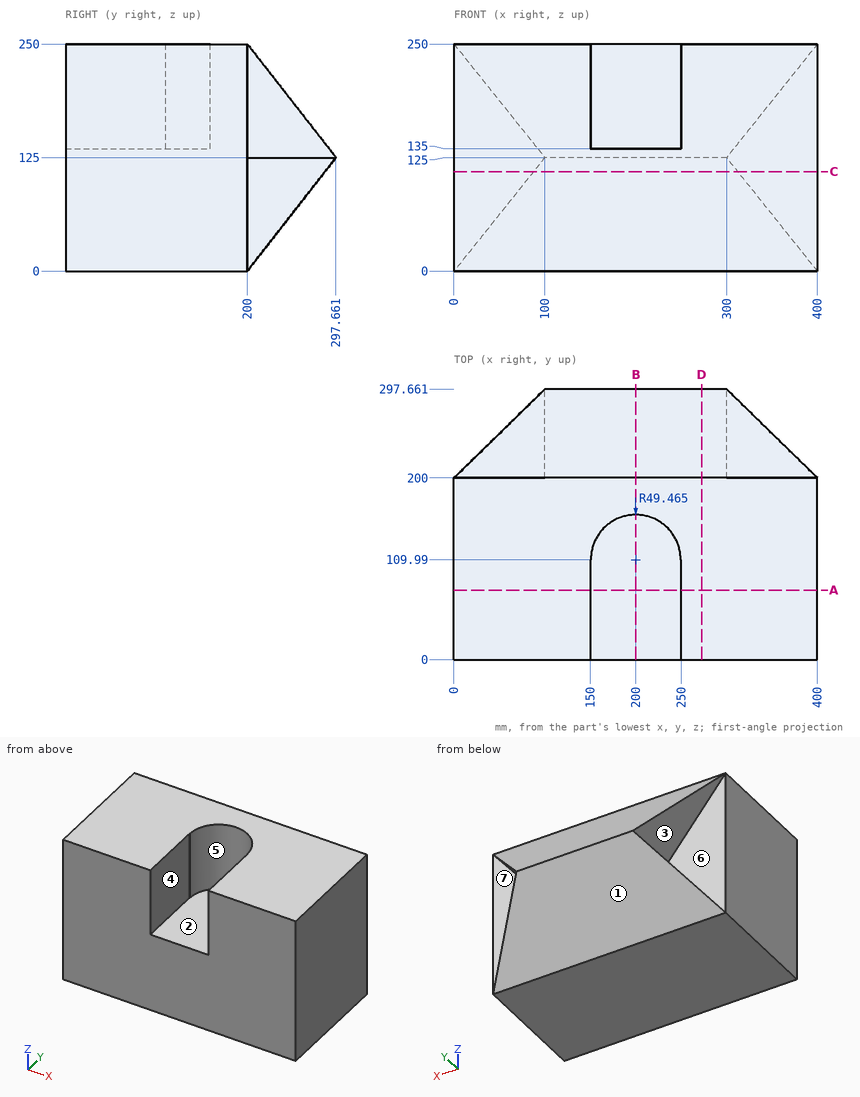
Part print with two shaded views. Sizes in mm from the minimum x, y, z corner. A direction names the side the tool comes from. Round coordinates to 2 decimals unless told otherwise and drop trailing zeros. Order: outer loops, then holes, each group sorted by start corner. A loop starts at its lowest first (then second) coordinate and runs counter-clockwise, first axis right, second up. Notation, with made-up numbers: (24.5, 48.5) - (83.5, 48.5) arc R19 cw to (83.5, 63.5) - close; hole circle Ø3 at (76, -11). An arc over 180 degrees is marked (long way). Answer as CSV lines item,"result". Start each with the question number.
1. Saw through at D-D, the plane x = 272.5. Write the cut outline in (y, z), and give its area (3 significant figures).
2. Saw through at B-B, the plane x = 200. Write the cut outline in (y, z) (1 decimal).
3. Tool access for the marked faces 5, 6 and 7: list every direction of +Z, -Z, +X, -X, +Y, -Y with a clear straight run to the whole face (end or side of a thin tool).
4. Pin check, flat tips, straight feed: pin 1 (5 mm diameter, centred on y = 230, z = 149, fed in from -X); pin 2 (3 mm diameter, centred on x = 161, y = 259, fed in from -Z); pin 3 (3 mm diameter, centred on x = 238.5, z = 121.5, fed in from +Y). Stop position of each tip, or through.
5. Drill centre lines: L1, parallel to X at y = 65.5, z = 187; L2, parallel to Z at x = 84, y = 220; L3, parallel to Y at x = 20.5, z = 221. Where is each one in solid material? Low to high. Write a range as [from, to].
6. Saw through at A-A, the plane y = 76.5. Write the cut outline in (x, z), and give its area (3 significant figures).
7. Saw through at C-C, the plane z = 109.5. Write the cut outline in (x, y).
8. Pull direction X, two halves, no side cores. Call the marked faces 1, 2, 3 and 4: +X half, -X half, draft (parallel to the pull), parting line (faces both ways), or undercut.
Model answer:
1,outline,"(0, 0) - (200, 0) - (297.66, 125) - (200, 250) - (0, 250) - close"
1,area,"62,200 mm²"
2,outline,"(0, 0) - (200, 0) - (297.7, 125) - (200, 250) - (159.5, 250) - (159.5, 135) - (0, 135) - close"
3,face 5,"+Z, -Y"
3,face 6,"-X, +Y"
3,face 7,"+X, +Y"
4,pin 1,"stops at x = 78.8"
4,pin 2,"stops at z = 73.6"
4,pin 3,"stops at y = 296.1"
5,L1,"x = [0, 150], [250, 400]"
5,L2,"z = [25.6, 105], [145, 224.4]"
5,L3,"y = [0, 200]"
6,outline,"(0, 0) - (400, 0) - (400, 250) - (250, 250) - (250, 135) - (150, 135) - (150, 250) - (0, 250) - close"
6,area,"88,500 mm²"
7,outline,"(0, 0) - (400, 0) - (400, 200) - (312.4, 200) - (312.4, 285.55) - (87.6, 285.55) - (87.6, 200) - (0, 200) - close"
8,face 1,"draft"
8,face 2,"undercut"
8,face 3,"-X half"
8,face 4,"undercut"
